Geometry check sheet. Reference: the model listing, model coordinates, mm. Give positions to 0.01 mm unless a question says otherwise; leave off trailing zeros. Write each loop counter-clockwise with the first axis right and the second up, starting at its lowest first coordinate (ties: lowest second). Pieces come first, ordered by that corner, then holes.
(1) Mould release check, pull along Z, two halves, no side actions. Record for faces 1 (the cylindrical face through (-2.53, 0.68, -0.05)), 2 (the flat face through (0, 1, 4)), 3 (the cylindrical face through (4.97, 0.68, -0.05)), 4 (the flat face through (-7.5, 1, 0)): +Z half, -Z half, draft (parallel to the pull), parting line (faces both ways), or undercut.
(2) Cross-section at C-C (y = 0.5). Record the boundary of the cut face in (x, z), and give its area (3 significant figures).
(3) Thickness scan on line 1 along Z through (x, y) = (3.75, 0.95); line 2 along X through (y, z) = (1.1, -1); line 3 along X through (y, z) = (0.7, 0.25). Record the ranges inside material, lowest first.
(4) Cross-section at A-A (z = 0). Record the boundary of the cut face in (x, y), and give its area (3 significant figures).
(5) Cross-section at B-B (x = 3.75). Record the boundary of the cut face in (y, z), and give its area (3 significant figures).
```python
from build123d import *

# Parameters (mm, degrees)
SKETCH1_W                       = 15
SKETCH1_H                       = 8
BOSS_EXTRUDE1_DEPTH             = 1.5875
F_2_CLEARANCE_HOLE1_D           = 2.4384
F_2_CLEARANCE_HOLE1_DEPTH       = 64.75
F_2_CLEARANCE_HOLE1_CSINK_D     = 2.794
F_2_CLEARANCE_HOLE1_CSINK_ANGLE = 82
F_2_CLEARANCE_HOLE1_TIP         = 0.732569267


with BuildPart() as part:
    # Sketch1 → Boss-Extrude1 (new body)
    with BuildSketch(Plane(origin=(0, 0, 0), x_dir=(1, 0, 0), z_dir=(0, 1, 0))):
        Rectangle(SKETCH1_W, SKETCH1_H)
    extrude(amount=BOSS_EXTRUDE1_DEPTH)

    # #2 Clearance Hole1
    with Locations(Plane(origin=(0, 1.5875, 0), x_dir=(1, 0, 0), z_dir=(0, 1, 0))):
        with Locations((-3.75, 0), (3.75, 0)):
            CounterSinkHole(F_2_CLEARANCE_HOLE1_D / 2, F_2_CLEARANCE_HOLE1_CSINK_D / 2, depth=F_2_CLEARANCE_HOLE1_DEPTH, counter_sink_angle=F_2_CLEARANCE_HOLE1_CSINK_ANGLE)
            with Locations((0, 0, -(F_2_CLEARANCE_HOLE1_DEPTH + F_2_CLEARANCE_HOLE1_TIP / 2))):  # 118° drill point
                Cone(0, F_2_CLEARANCE_HOLE1_D / 2, F_2_CLEARANCE_HOLE1_TIP, mode=Mode.SUBTRACT)


solid = part.part
```
Reply:
1. face 1: undercut
1. face 2: +Z half
1. face 3: undercut
1. face 4: draft
2. outline: (-7.5, -4) - (7.5, -4) - (7.5, 4) - (-7.5, 4) - close; hole circle Ø2.44 at (-3.75, 0); hole circle Ø2.44 at (3.75, 0)
2. area: 111 mm2
3. line 1: z = -4 to -1.22, 1.22 to 4
3. line 2: x = -7.5 to -4.45, -3.05 to 3.05, 4.45 to 7.5
3. line 3: x = -7.5 to -4.94, -2.56 to 2.56, 4.94 to 7.5
4. outline: (-7.5, 0) - (-4.97, 0) - (-4.97, 1.38) - (-5.15, 1.59) - (-7.5, 1.59) - close; (-2.53, 0) - (2.53, 0) - (2.53, 1.38) - (2.35, 1.59) - (-2.35, 1.59) - (-2.53, 1.38) - close; (4.97, 0) - (7.5, 0) - (7.5, 1.59) - (5.15, 1.59) - (4.97, 1.38) - close
4. area: 16.0 mm2
5. outline: (0, -4) - (1.59, -4) - (1.59, -1.4) - (1.38, -1.22) - (0, -1.22) - close; (0, 1.22) - (1.38, 1.22) - (1.59, 1.4) - (1.59, 4) - (0, 4) - close
5. area: 8.79 mm2
